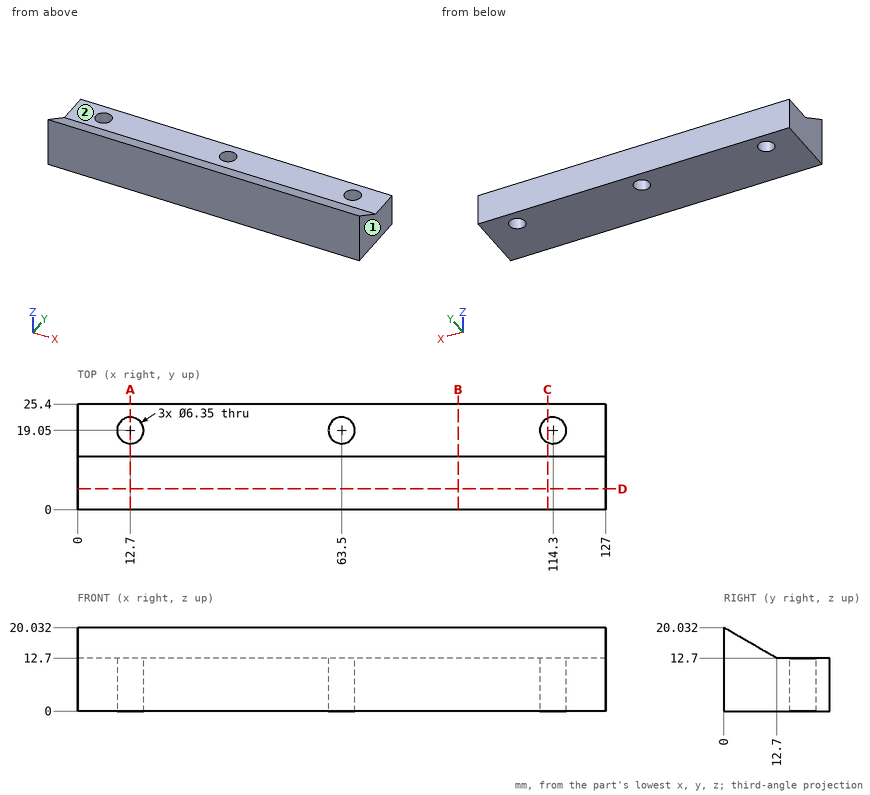
Drawing for the job (mm, zero at the part's lowest x, y, z). A direction names the side the tool comes from. Round coordinates to 2 decimals unless told otherwise and drop trailing zeros. Write each loop counter-clockwise with the first axis right and the second up, starting at its lowest first coordinate (ties: lowest second). Pieces come first, ordered by that corner, then holes. Notation, with made-up numbers: M 82,17.25 L 91,17.25 A24 cw 91,30.25 Z; hole C 14.25,27.25 d4. An arc over 180 degrees is marked long. Put each result on its own line as item: value.
Item 1: Flat gauge pins, fed straight in: P1, Ø8, axis at x = 95.5, y = 5, coming from the +Z side (1 decimal); P2, Ø10, axis at x = 12.7, y = 19.05, coming from the +Z side; P3, Ø5, axis at x = 114.3, y = 19.05, coming from the +Z side. Where does each tip first touch, or does it go through?
Responses:
P1: z = 19.5
P2: z = 12.7
P3: through
Item 2: Cut at B-B (x = 91.5). List the corners of the cut face in (y, z).
Responses:
outline: M 0,0 L 25.4,0 L 25.4,12.7 L 12.7,12.7 L 0,20.03 Z
Item 3: Cut at A-A (x = 12.7). List the corners of the cut face in (y, z) (1 decimal).
Responses:
outline: M 0,0 L 15.9,0 L 15.9,12.7 L 12.7,12.7 L 0,20 Z; M 22.2,0 L 25.4,0 L 25.4,12.7 L 22.2,12.7 Z
Item 4: Cut at C-C (x = 113). List the corners of the cut face in (y, z).
Responses:
outline: M 0,0 L 16.15,0 L 16.15,12.7 L 12.7,12.7 L 0,20.03 Z; M 21.95,0 L 25.4,0 L 25.4,12.7 L 21.95,12.7 Z
Item 5: Tool access for the marked faces 1 and 2: list every direction of +Z, -Z, +X, -X, +Y, -Y with a clear straight run to the whole face (end or side of a thin tool).
Responses:
face 1: +Z, -Z, +X, +Y, -Y
face 2: +Z, +X, -X, +Y
Item 6: Cut at D-D (y = 5). List the corners of the cut face in (x, z) (1 decimal), and give its area (3 significant figures).
Responses:
outline: M 0,0 L 127,0 L 127,17.1 L 0,17.1 Z
area: 2,180 mm²
Item 7: Probe L1, parallel to X at y = 19.05, z = 8.5 (1 decimal); L2, parallel to Y at x = 63.5, z = 3.75 (1 decimal); L3, parallel to Z at x = 9, y = 19.5. List the from-to ranges inside material, lowest first. Write a range as from..to.
Responses:
L1: 0..9.5, 15.9..60.3, 66.7..111.1, 117.5..127
L2: 0..15.9, 22.2..25.4
L3: 0..12.7
